from build123d import *

# Parameters (mm, degrees)
F0_W     = 102
F0_H     = 40
F1_DEPTH = 3
F2_W     = 3
F2_H     = 5
F3_DEPTH = 3
F4_W     = 5
F4_H     = 3
F5_DEPTH = 3


with BuildPart() as f1:
    # F0 (on Front) → F1 (new body)
    with BuildSketch(Plane.XZ):
        Rectangle(F0_W, F0_H)
    extrude(amount=F1_DEPTH)

    # F2 (on face) → F3 (join)
    with BuildSketch(Plane.XZ.offset(3)):
        with Locations((-52.5, -17.5)):
            Rectangle(F2_W, F2_H)
        with Locations((-52.5, -7.5)):
            Rectangle(F2_W, F2_H)
        with Locations((-52.5, 2.5)):
            Rectangle(F2_W, F2_H)
        with Locations((-52.5, 12.5)):
            Rectangle(F2_W, F2_H)
        with Locations((52.5, -7.5)):
            Rectangle(F2_W, F2_H)
        with Locations((52.5, -17.5)):
            Rectangle(F2_W, F2_H)
        with Locations((52.5, 12.5)):
            Rectangle(F2_W, F2_H)
        with Locations((52.5, 2.5)):
            Rectangle(F2_W, F2_H)
    extrude(amount=-F3_DEPTH)

    # F4 (on face) → F5 (join)
    with BuildSketch(Plane.XZ.offset(3)):
        with Locations((5, -21.5)):
            Rectangle(F4_W, F4_H)
        with Locations((15, -21.5)):
            Rectangle(F4_W, F4_H)
        with Locations((25, -21.5)):
            Rectangle(F4_W, F4_H)
        with Locations((35, -21.5)):
            Rectangle(F4_W, F4_H)
        with Locations((45, -21.5)):
            Rectangle(F4_W, F4_H)
        with Locations((-25, -21.5)):
            Rectangle(F4_W, F4_H)
        with Locations((-15, -21.5)):
            Rectangle(F4_W, F4_H)
        with Locations((-5, -21.5)):
            Rectangle(F4_W, F4_H)
        with Locations((-35, -21.5)):
            Rectangle(F4_W, F4_H)
        with Locations((-45, -21.5)):
            Rectangle(F4_W, F4_H)
    extrude(amount=-F5_DEPTH)


solid = f1.part
Work out the finished part from the listing and answer in its coordinate system (mm). A direction names the side the tool comes from. Give positions to 0.01 mm unless a question says otherwise; leave off trailing zeros. Write each loop counter-clockwise with the first axis right and the second up, starting at its lowest first coordinate (ties: lowest second). Pieces come first, ordered by that corner, then holes. Notation, with made-up numbers: (82.25, -5) - (111.25, -5) arc R21 ccw to (111.25, 33) - close; hole circle Ø6 at (-14, 80.25). An arc over 180 degrees is marked (long way). One line per item, written item: value. Start each with the question number.
1. Find section B-B (x = -1.5). Write down the section's boundary in (y, z).
2. Consider probe 1 along Z at (x, y) = (-8, -1.05); probe 2 along X at (y, z) = (-2.5, 8.5). Determine where each line is inside the solid, lowest interval first.
3. Given pin 1 (1.5 mm diameter, centred on y = -1, z = 18.5, fed in from -X); pin 2 (1.5 mm diameter, centred on x = 19, y = -1.5, fed in from -Z); pin 3 (1.5 mm diameter, centred on y = -1.5, z = -22, fed in from -X), each flat-ended and moving along its own axis, determine where each tip first touches the part or whether it passes through.
4. For a pull along Z with two mould halves and no side action, classify faces 5 (the flat face through (-53, -2, 0)), 6 (the flat face through (-20, -2, -20)), 7 (the flat face through (22.5, -2, -22)), 8 (the flat face through (51, -1, -3)) as +Z half, -Z half, draft (parallel to the pull), parting line (faces both ways), or undercut.
5. Find section A-A (z = -4). Write down the section's boundary in (x, y), then the cut area to 3 significant figures.
6. For faces 1 (the flat face through (52, -2, 15)), 2 (the flat face through (10, -2, -20)), 3 (the flat face through (-53, -2, 15)), 4 (the flat face through (-53, -2, -10)), determine the directions among +Z, -Z, +X, -X, +Y, -Y from which every point of the face is accessible in a straight line to the end or side of a thin tool.
Geometry results:
1. outline: (-3, -20) - (0, -20) - (0, 20) - (-3, 20) - close
2. probe 1: -20 to 20
2. probe 2: -51 to 51
3. pin 1: x = -51
3. pin 2: z = -20
3. pin 3: x = -47.5
4. face 5: undercut
4. face 6: -Z half
4. face 7: draft
4. face 8: undercut
5. outline: (-51, -3) - (51, -3) - (51, 0) - (-51, 0) - close
5. area: 306 mm2
6. face 1: +Z, +X, +Y, -Y
6. face 2: -Z, +Y, -Y
6. face 3: +Z, -X, +Y, -Y
6. face 4: -X, +Y, -Y
